```python
from build123d import *

# Parameters (mm, degrees)
SKETCH2_W                = 41
SKETCH2_H                = 41
BOSS_EXTRUDE1_DEPTH      = 3
SKETCH3_R                = 1
CUT_EXTRUDE1_DEPTH       = 0.2
SKETCH4_R                = 0.6
CUT_EXTRUDE2_DEPTH       = 41
SKETCH5_R                = 0.6
CUT_EXTRUDE3_DEPTH       = 41
SKETCH6_R                = 0.6
BOSS_EXTRUDE2_DEPTH      = 25
BOSS_EXTRUDE2_DEPTH_BACK = 1


with BuildPart() as part:
    # Sketch2 → Boss-Extrude1 (new body)
    with BuildSketch(Plane(origin=(0, 0, 0), x_dir=(1, 0, 0), z_dir=(0, 1, 0))):
        Rectangle(SKETCH2_W, SKETCH2_H)
    extrude(amount=BOSS_EXTRUDE1_DEPTH)

    # Sketch3 → Cut-Extrude1 (cut)
    with BuildSketch(Plane.ZY.offset(20.5)):
        with Locations((-18.087798173, 1.496190707)):
            Circle(SKETCH3_R)
        with Locations((18.087798173, 1.496190707)):
            Circle(SKETCH3_R)
    extrude(amount=-CUT_EXTRUDE1_DEPTH, mode=Mode.SUBTRACT)

    # Sketch4 → Cut-Extrude2 (cut)
    with BuildSketch(Plane.ZY.offset(20.5)):
        with Locations((-20.5, 1.5)):
            Circle(SKETCH4_R)
        with Locations((20.5, 1.5)):
            Circle(SKETCH4_R)
    extrude(amount=-CUT_EXTRUDE2_DEPTH, mode=Mode.SUBTRACT)

    # Sketch5 → Cut-Extrude3 (cut)
    with BuildSketch(Plane.XY.offset(20.5)):
        with Locations((-20.5, 1.5)):
            Circle(SKETCH5_R)
        with Locations((20.5, 1.5)):
            Circle(SKETCH5_R)
    extrude(amount=-CUT_EXTRUDE3_DEPTH, mode=Mode.SUBTRACT)

    # Sketch6 → Boss-Extrude2 (add, two sides)
    with BuildSketch(Plane.ZY.offset(20.5)) as boss_extrude2_sk:
        with Locations((-18.087798173, 1.496190707)):
            Circle(SKETCH6_R)
        with Locations((18.087798173, 1.496190707)):
            Circle(SKETCH6_R)
    extrude(amount=BOSS_EXTRUDE2_DEPTH)
    extrude(boss_extrude2_sk.sketch, amount=-BOSS_EXTRUDE2_DEPTH_BACK)


solid = part.part
```
Here's how the part is built. I have some questions about the finished solid (model axes, mm). A direction names the side the tool comes from. Give positions to 0.01 mm unless a question says otherwise; leave off trailing zeros. Order: outer loops, then holes, each group sorted by start corner. A loop starts at its lowest first (then second) coordinate and runs counter-clockwise, first axis right, second up. Notation, with made-up numbers: M 9.25,29.25 L 29.25,29.25 A28 cw 29.25,63.25 Z; hole C 33.25,65 d1. An arc over 180 degrees is marked long. Use a Markdown table: item, result. Add a question column.
1. Suppose I cut it at A-A (z = -14). List the corners of the cut face in (x, y) for me.
2. I need wall thicknesses on probe 1 along X at (y, z) = (0.7, -2); probe 2 along Z at (x, y) = (-23, 1.65); probe 3 along Z at (x, y) = (-33, 1.75). Which ranges of each line are inside material? Lowest first, please. Write a range as from..to.
3. On a 3-axis mill with a long thin cutter (end or side, diameter ignored), from which of +Z, -Z, +X, -X, +Y, -Y can I reach the whole of each face in a straight line? I mean faces 4 (the flat face through (0, 3, 0)), 5 (the cylindrical face through (-32.88, 1.27, -17.53)). Say none if no direction works.
4. If we mould it in two halves opening along Z, with no side actions, what happens to faces 1 (the cylindrical face through (-0.3, 1.5, 19.9)), 2 (the flat face through (-45.5, 1.5, -18.1)), 3 (the cylindrical face through (-32.879, 1.266, 18.642))? For each: +Z half, -Z half, draft (parallel to the pull), parting line (faces both ways), or undercut.
5. Suppose I cut it at B-B (x = -38). List the corners of the cut face in (y, z) for me.
6. For pin 1 Ø0.5 at (y, z) = (2.5, 7) entering from -X, with a flat end and sliding along its axis, tell me the tip position at first contact or that it passes through.
Results list:
| question | item | result |
|---|---|---|
| 1 | outline | M -20.5,0 L 20.5,0 L 20.5,0.9 A0.6 cw 20.5,2.1 L 20.5,3 L -20.5,3 L -20.5,2.1 A0.6 cw -20.5,0.9 Z |
| 2 | probe 1 | x = -20.5..20.5 |
| 2 | probe 2 | z = -18.67..-17.51, 17.51..18.67 |
| 2 | probe 3 | z = -18.63..-17.54, 17.54..18.63 |
| 3 | face 4 | +Z, -Z, +X, -X, +Y |
| 3 | face 5 | -X |
| 4 | face 1 | +Z half |
| 4 | face 2 | draft |
| 4 | face 3 | undercut |
| 5 | outline | C 1.5,-18.09 d1.2; C 1.5,18.09 d1.2 |
| 6 | pin 1 | stops at x = -20.5 |
